Part print with two shaded views. Sizes in mm from the minimum x, y, z corner. Give positions to 0.01 mm unless a question says otherwise; leave off trailing zeros. Write each loop counter-clockwise with the first axis right and the second up, starting at its lowest first coordinate (ties: lowest second). Pieces come first, ordered by that corner, then holes. Notation, with made-up numbers: (85, 54) -> (133, 54) arc R5 ccw to (133, 58) -> close; hole circle Ø4 at (-31, 77.25). An arc over 180 degrees is marked (long way). Answer as a JSON object with one key per item and string values.
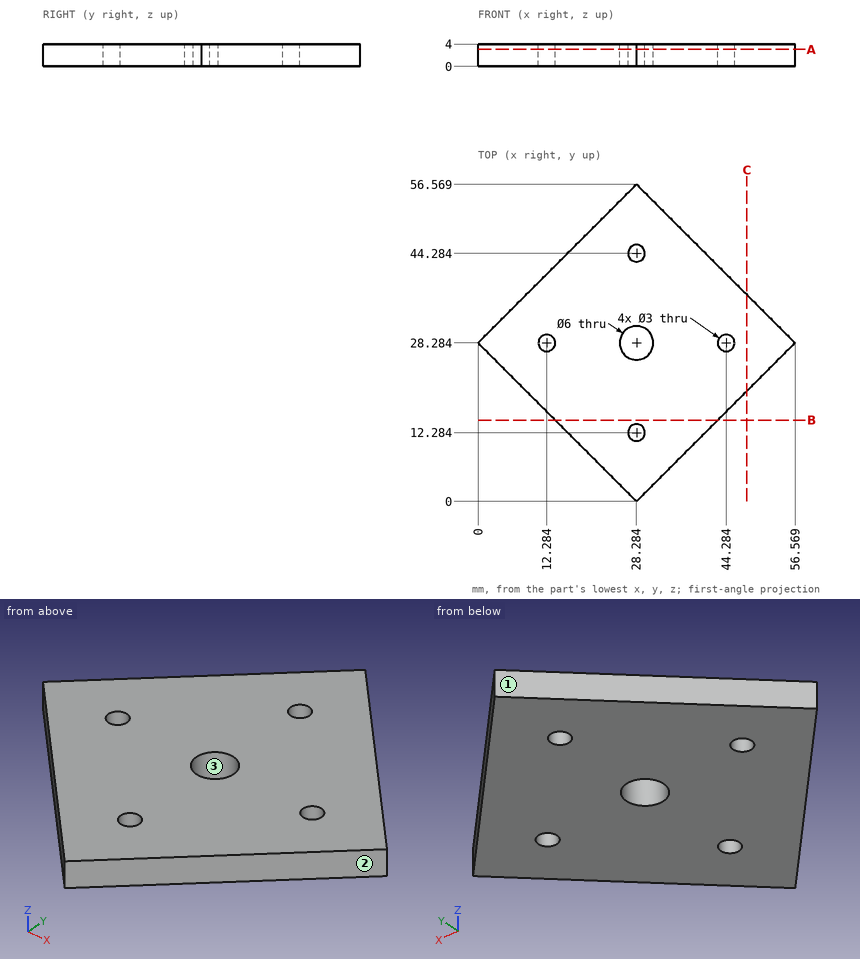
1) Slice it at A-A (z = 3.05). List the corners of the cut face in (x, y) (1 decimal).
Model answer:
{"outline": "(0, 28.3) -> (28.3, 0) -> (56.6, 28.3) -> (28.3, 56.6) -> close; hole circle Ø3 at (12.3, 28.3); hole circle Ø6 at (28.3, 28.3); hole circle Ø3 at (28.3, 12.3); hole circle Ø3 at (28.3, 44.3); hole circle Ø3 at (44.3, 28.3)"}
2) Slice it at B-B (y = 14.5). List the corners of the cut face in (x, z) (1 decimal).
Model answer:
{"outline": "(13.8, 0) -> (42.8, 0) -> (42.8, 4) -> (13.8, 4) -> close"}
3) Slice it at C-C (x = 48). List the corners of the cut face in (y, z) (1 decimal).
Model answer:
{"outline": "(19.7, 0) -> (36.9, 0) -> (36.9, 4) -> (19.7, 4) -> close"}
4) Mould opens along X. For the marked faces 1, 2 and 3 say: released by +X, released by -X, zero draft, split by the parting line, or undercut.
Model answer:
{"face 1": "released by -X", "face 2": "released by +X", "face 3": "undercut"}
5) Pin check, flat tips, straight feed: pin 1 (2 mm diameter, centred on x = 41.5, z = 1, fed in from +Y); pin 2 (1 mm diameter, centred on x = 32, z = 2, fed in from +Y). Stop position of each tip, or through.
Model answer:
{"pin 1": "stops at y = 44.35", "pin 2": "stops at y = 53.35"}
6) Wall check: probe 1 along Y at (x, z) = (3, 2.5) (1 decimal); probe 2 along Y at (x, z) = (11, 0.3) (1 decimal); probe 3 along X at (y, z) = (28, 2.15) (1 decimal). Give the ranges that are in metal, low to high.
Model answer:
{"probe 1": "y = 25.3 to 31.3", "probe 2": "y = 17.3 to 27.5, 29.1 to 39.3", "probe 3": "x = 0.3 to 10.8, 13.8 to 25.3, 31.3 to 42.8, 45.8 to 56.3"}
